Read the model definition and answer for the solid it produces. Units are mm, in the model's axes. A direction names the side the tool comes from. Give positions to 0.01 mm unless a question says otherwise; leave off trailing zeros. Write each loop counter-clockwise with the first axis right and the second up, starting at its lowest first coordinate (ties: lowest second). Pieces come first, ordered by that corner, then holes. Notation, with made-up numbers: (-13.75, 36.25) -> (0.25, 36.25) arc R15 cw to (0.25, 43.25) -> close; hole circle Ø5 at (-21, 84). An arc over 180 degrees is marked (long way). Use a Markdown table: item, result.
from build123d import *

# Parameters (mm, degrees)
F0_W         = 65
F0_H         = 65
F1_DEPTH     = 4
F3_DEPTH     = 60
F5_DEPTH     = 105.7
F7_DEPTH     = 25
F8_T4_DEPTH  = 26.0981202527
F8_T10_DEPTH = 26.0981202527
F9_SIZE      = 2
F10_DEPTH    = 20
F11_DEPTH    = 3
F12_DEPTH    = 3
F14_DEPTH    = 5
F15_DEPTH    = 15
F16_DEPTH    = 15
F18_DEPTH    = 71
F19_R        = 9.99999
F20_R        = 12.99999


# Not quite as in the source:
# - a fillet or chamfer that OpenCascade refuses, or shapes differently, is made with other operations: its cross-section is extruded or revolved along the edge and cut away or added
# - a fillet or chamfer is up to 0.001 mm smaller than in the source, because OpenCascade refuses the exact size


with BuildPart() as f1:
    # F0 (on Top) → F1 (new body)
    with BuildSketch(Plane.XY):
        Rectangle(F0_W, F0_H)
        Polygon((32.5, -32.5), (-32.5, -32.5), (-32.5, 32.5), (-35.5, 32.5), (-35.5, -35.5), (0, -35.5), (35.5, -35.5), (35.5, 32.5), (32.5, 32.5), align=None)
        Polygon((0, -35.5), (-35.5, -35.5), (-35.5, -50.5), (-5, -50.5), align=None)
        Polygon((-35.5, -50.5), (-35.5, -35.5), (-50.5, -50.5), align=None)
        Polygon((35.5, -50.5), (35.5, -35.5), (0, -35.5), (5, -50.5), (5.9827403165, -50.5), align=None)
        Polygon((50.5, -50.5), (35.5, -35.5), (35.5, -50.5), align=None)
    extrude(amount=F1_DEPTH)

    # F2 (on face) → F3 (join)
    with BuildSketch(Plane.XY.offset(4)):
        Polygon((32.5, -32.5), (-32.5, -32.5), (-32.5, 32.5), (-35.5, 32.5), (-35.5, -35.5), (0, -35.5), (35.5, -35.5), (35.5, 32.5), (32.5, 32.5), align=None)
    extrude(amount=F3_DEPTH)

    # F4 (on face) → F5 (cut)
    with BuildSketch(Plane.YZ.offset(35.5)):
        Polygon((-32.5, 64), (32.5, 4), (32.5, 64), align=None)
    extrude(amount=-F5_DEPTH, mode=Mode.SUBTRACT)

    # F6 (on face) → F7 (cut)
    with BuildSketch(Plane.XZ.offset(35.5)):
        Polygon((-5, 8), (0, 8), (3.482630942, 8), (25, 8), (25, 19), (5, 19), (5, 37), (0, 37), (-5, 37), (-5, 19), (-25, 19), (-25, 8), align=None)
    extrude(amount=-F7_DEPTH, mode=Mode.SUBTRACT)

    # F8: chamfer of 2 on 1 edges, made by hand


with BuildPart() as f8_tool2:
    # F8_s3 → F8_t4 (new body)
    with BuildSketch(Plane(origin=(-17.2764751324, -51.8294253971, 0), x_dir=(0, 0, 1), z_dir=(0.316227766, 0.9486832981, 0))):
        Polygon((2, 11.2260856936), (4, 9.2260856936), (4, 11.2260856936), align=None)
    extrude(amount=F8_T4_DEPTH)

    split(bisect_by=Plane.XZ.offset(35.5), keep=Keep.TOP)

    split(bisect_by=Plane(origin=(-10.65, -3.55, 0), x_dir=(0, 0, 1), z_dir=(-0.9486832981, -0.316227766, 0)), keep=Keep.TOP)


with BuildPart() as f1_1:
    add(f1.part)

    # F8_t1: cut F8_tool2
    add(f8_tool2.part, mode=Mode.SUBTRACT)


with BuildPart() as f8_tool8:
    # F8_s9 → F8_t10 (new body)
    with BuildSketch(Plane(origin=(-17.2764751324, -51.8294253971, 0), x_dir=(0, 0, 1), z_dir=(0.316227766, 0.9486832981, 0))):
        Polygon((2, 11.2260856936), (4, 9.2260856936), (4, 11.2260856936), align=None)
    extrude(amount=F8_T10_DEPTH)

    split(bisect_by=Plane.XZ.offset(32.5), keep=Keep.BOTTOM)

    split(bisect_by=Plane(origin=(-10.65, -3.55, 0), x_dir=(0, 0, 1), z_dir=(-0.9486832981, -0.316227766, 0)), keep=Keep.TOP)


with BuildPart() as f1_2:
    add(f1_1.part)

    # F8_t7: cut F8_tool8
    add(f8_tool8.part, mode=Mode.SUBTRACT)

    # F9
    f9_edges = [f1_2.edges().sort_by_distance(p)[0] for p in [
        (2.5, -43, 4),
    ]]
    chamfer(f9_edges, length=F9_SIZE)

    # F10 (add): a face of the model
    f10_faces = [f1_2.faces().sort_by_distance(p)[0] for p in [
        (0, 32.5, 2),
    ]]
    extrude(f10_faces, amount=F10_DEPTH)

    # F11 (add): a face of the model
    f11_faces = [f1_2.faces().sort_by_distance(p)[0] for p in [
        (15, -34, 19),
    ]]
    extrude(f11_faces, amount=-F11_DEPTH)

    # F12 (add): a face of the model
    f12_faces = [f1_2.faces().sort_by_distance(p)[0] for p in [
        (-15, -34, 19),
    ]]
    extrude(f12_faces, amount=-F12_DEPTH)

    # F13 (on face) → F14 (join)
    with BuildSketch(Plane(origin=(0, -32.5, 0), x_dir=(-1, 0, 0), z_dir=(0, 1, 0))):
        Polygon((32.5, 8), (25, 8), (-25, 8), (-32.5, 8), (-32.5, 4), (1, 4), (1, 3.8973665961), (1.1081851068, 4), (32.5, 4), align=None)
    extrude(amount=F14_DEPTH)

    # F15 (add): a face of the model
    f15_faces = [f1_2.faces().sort_by_distance(p)[0] for p in [
        (15, -34, 19),
    ]]
    extrude(f15_faces, amount=F15_DEPTH)

    # F16 (add): a face of the model
    f16_faces = [f1_2.faces().sort_by_distance(p)[0] for p in [
        (-15, -34, 19),
    ]]
    extrude(f16_faces, amount=F16_DEPTH)

    # F17 (on face) → F18 (join)
    with BuildSketch(Plane(origin=(-35.5, 0, 0), x_dir=(0, -1, 0), z_dir=(-1, 0, 0))):
        Polygon((32.5, 74), (32.5, 64), (35.5, 64), (35.5, 77), (22.5, 77), (22.5, 74), align=None)
    extrude(amount=-F18_DEPTH)

    # F19 (radius 10 in the source; OpenCascade refuses exactly that, so slightly less here)
    f19_edges = [f1_2.edges().sort_by_distance(p)[0] for p in [
        (0, -32.5, 74),
    ]]
    fillet(f19_edges, radius=F19_R)

    # F20 (radius 13 in the source; OpenCascade refuses exactly that, so slightly less here)
    f20_edges = [f1_2.edges().sort_by_distance(p)[0] for p in [
        (0, -35.5, 77),
    ]]
    fillet(f20_edges, radius=F20_R)


solid = f1_2.part
Item 1: A cutting plane is placed at A-A (z = 20). Give the vertices of the cut face in (x, y).
Return value:
| item | result |
|---|---|
| outline | (-35.5, -35.5) -> (-5, -35.5) -> (-5, -32.5) -> (-32.5, -32.5) -> (-32.5, 15.17) -> (-35.5, 15.17) -> close; (5, -35.5) -> (35.5, -35.5) -> (35.5, 15.17) -> (32.5, 15.17) -> (32.5, -32.5) -> (5, -32.5) -> close |
Item 2: Each of these flat-tipped pins is pushed along its axis until it touches: P1, Ø7.5, axis at x = 20.5, y = -46, coming from the +Z side; P2, Ø1.5, axis at y = -33.5, z = 28, coming from the -X side; P3, Ø12, axis at x = -35.5, y = 35, coming from the +Z side. Where does it stop, or does it pass through?
Return value:
| item | result |
|---|---|
| P1 | z = 4 |
| P2 | x = -35.5 |
| P3 | z = 7.23 |
Item 3: A cutting plane is placed at B-B (y = -37). Give the vertices of the cut face in (x, z), then the cut area to 3 significant figures.
Return value:
| item | result |
|---|---|
| outline | (-37, 0) -> (-0.5, 0) -> (-0.5, 2) -> (-2.61, 4) -> (-37, 4) -> close; (0.5, 0) -> (37, 0) -> (37, 4) -> (2.61, 4) -> (0.5, 2) -> close |
| area | 288 mm^2 |
Item 4: For a pull along Z with two mould halves and no side action, classify faces 1 (the face through (-28, -50.5, 2)), 2 (the face through (-32.5, -8, 27)), 3 (the face through (1, 0, 0)), 4 (the face through (32.5, -14, 20)) as +Z half, -Z half, draft (parallel to the pull), parting line (faces both ways), or undercut.
Return value:
| item | result |
|---|---|
| face 1 | draft |
| face 2 | undercut |
| face 3 | -Z half |
| face 4 | undercut |
Item 5: A tool of negligible diameter and unlimited length cuts with its end or side. For faces 5 (the face through (26, -43, 4)), 6 (the face through (-2.535, -43.105, 0.986)), 7 (the face through (0, -31, 8)), 8 (the face through (3.504, -42.895, 2.986)), from which of +Z, -Z, +X, -X, +Y, -Y can it reach the whole face along a straight path? Write none if from no direction.
Return value:
| item | result |
|---|---|
| face 5 | +Z, +X, -X, -Y |
| face 6 | +Z, -Z, -Y |
| face 7 | +Y |
| face 8 | +Z, -Y |
Item 6: A cutting plane is placed at D-D (y = 15.5). Give the vertices of the cut face in (x, z).
Return value:
| item | result |
|---|---|
| outline | (-35.5, 0) -> (35.5, 0) -> (35.5, 19.69) -> (32.5, 19.69) -> (32.5, 4) -> (-32.5, 4) -> (-32.5, 19.69) -> (-35.5, 19.69) -> close |
Item 7: Straight lines are drawn through the part: line 1 along X through (y, z) = (9, 23); line 2 along Z through (x, y) = (9.5, -21.5); line 3 along X through (y, z) = (-35, 11). For each, find the intervals that lie inside material, in ascending order. Write a range as [from, to].
Return value:
| item | result |
|---|---|
| line 1 | [-35.5, -32.5], [32.5, 35.5] |
| line 2 | [0, 4] |
| line 3 | [-35.5, -5], [5, 35.5] |
